Model file for the job. Use its own axes, mm. Give positions to 0.01 mm unless a question says otherwise; leave off trailing zeros. Loops run counter-clockwise (first coordinate to the right, second up) from the corner with the lowest first, then second, coordinate; pieces in that order, holes last. Notation, with made-up numbers: M 62.25,44 L 86.25,44 A38 ccw 86.25,82 Z; hole C 83,-32.5 d2. An arc over 180 degrees is marked long. Answer in a Markdown table with one row per item.
```python
from build123d import *

# Parameters (mm, degrees)
F1_DEPTH = 2
F2_SIZE  = 1
F3_R     = 3.5
F4_DEPTH = 10
F5_R     = 1.5
F6_DEPTH = 15


with BuildPart() as f1:
    # F0 (on Top) → F1 (new body)
    with BuildSketch(Plane.XY):
        Polygon((-30, 0), (0, 0), (50, 0), (50, 40), (0, 40), (-30, 22), align=None)
    extrude(amount=F1_DEPTH)

    # F2
    f2_edges = [f1.edges().sort_by_distance(p)[0] for p in [
        (10, 0, 2),
        (-30, 11, 2),
        (-15, 31, 2),
        (25, 40, 2),
        (50, 20, 2),
    ]]
    chamfer(f2_edges, length=F2_SIZE)

    # F3 (on face) → F4 (join)
    with BuildSketch(Plane.XY.offset(2)):
        with Locations((0.276984, 24)):
            Circle(F3_R)
    extrude(amount=F4_DEPTH)

    # F5 (on face) → F6 (cut)
    with BuildSketch(Plane.XY.offset(12)):
        with Locations((0.276984, 24)):
            Circle(F5_R)
    extrude(amount=-F6_DEPTH, mode=Mode.SUBTRACT)


solid = f1.part
```
Q1. Saw through at D-D (x = 34). Give the cut face in (y, z).
Reported:
| item | result |
|---|---|
| outline | M 0,0 L 40,0 L 40,1 L 39,2 L 1,2 L 0,1 Z |
Q2. Saw through at C-C (z = 5.75). Give the cut face in (x, y), and give its area (3 significant figures).
Reported:
| item | result |
|---|---|
| outline | C 0.28,24 d7; hole C 0.28,24 d3 |
| area | 31.4 mm² |
Q3. Saw through at B-B (y = 14.5). Give the cut face in (x, z), and give its area (3 significant figures).
Reported:
| item | result |
|---|---|
| outline | M -30,0 L 50,0 L 50,1 L 49,2 L -29,2 L -30,1 Z |
| area | 159 mm² |
Q4. Saw through at A-A (y = 24). Give the cut face in (x, z), and give its area (3 significant figures).
Reported:
| item | result |
|---|---|
| outline | M -26.67,0 L -1.22,0 L -1.22,12 L -3.22,12 L -3.22,2 L -24.72,2 L -26.67,1 Z; M 1.78,0 L 50,0 L 50,1 L 49,2 L 3.78,2 L 3.78,12 L 1.78,12 Z |
| area | 186 mm² |
Q5. Mould opens along Y. For faces 1 (the face through (0.082, 25.487, 6.084)), 2 (the face through (2, 24, 12)), 3 (the face through (-0.18, 27.47, 6.93)), 4 (the face through (-14.79, 31.126, 0.493)) say: released by +Y, released by -Y, zero draft, split by the parting line, or undercut.
Reported:
| item | result |
|---|---|
| face 1 | undercut |
| face 2 | zero draft |
| face 3 | split by the parting line |
| face 4 | released by +Y |
Q6. Drop a flat-ended pin along its axis: pin 1 (12 mm diameter, centred on x = -14, y = 19, fed in from +Z). Give the stop position or say it passes through.
Reported:
| item | result |
|---|---|
| pin 1 | z = 2 |
Q7. Probe probe 1 along Z at (x, y) = (4.5, 38). List the from-to ranges inside material, lowest first.
Reported:
| item | result |
|---|---|
| probe 1 | 0 to 2 |
